Source: CAD feature listing. Evaluate the final solid. Frame: model axes, mm. A direction names the side the tool comes from. Give positions to 0.01 mm unless a question says otherwise; leave off trailing zeros. Loops run counter-clockwise (first coordinate to the right, second up) from the corner with the lowest first, then second, coordinate; pieces in that order, holes last. Notation, with made-up numbers: (40.5, -31.5) - (83.5, -31.5) arc R30 cw to (83.5, 4.5) - close; hole circle Ø1 at (-25.75, 28.5). An arc over 180 degrees is marked (long way). Put each result on its own line as item: value.
```python
from build123d import *

# Parameters (mm, degrees)
SKETCH_1_R          = 4.5
EXTRUDE_1_DEPTH     = 10
EXTRUDE_2_DEPTH     = 9
EXTRUDE_3_DEPTH     = 14
CUT_EXTRUDE_1_DEPTH = 29


with BuildPart() as part:
    # 草圖1 → 填料-伸長1 (new body)
    with BuildSketch(Plane.XY):
        with BuildLine():
            Line((-36, 9), (36, 9))
            ThreePointArc((36, 9), (45, 0), (36, -9))
            Line((36, -9), (-36, -9))
            ThreePointArc((-36, -9), (-45, 0), (-36, 9))
        make_face()
        with Locations((36, 0)):
            Circle(SKETCH_1_R, mode=Mode.SUBTRACT)
        with Locations((-36, 0)):
            Circle(SKETCH_1_R, mode=Mode.SUBTRACT)
    extrude(amount=EXTRUDE_1_DEPTH)

    # 草圖3 → 填料-伸長2 (add, symmetric)
    with BuildSketch(Plane(origin=(0, 0, 0), x_dir=(1, 0, 0), z_dir=(0, 1, 0))):
        with BuildLine():
            Line((-30, 0), (30, 0))
            ThreePointArc((30, 0), (0, -30), (-30, 0))
        make_face()
    extrude(amount=EXTRUDE_2_DEPTH, both=True)

    # 草圖4 → 填料-伸長3 (add, symmetric)
    with BuildSketch(Plane(origin=(0, 0, 0), x_dir=(1, 0, 0), z_dir=(0, 1, 0))):
        with BuildLine():
            Line((-24, 0), (24, 0))
            ThreePointArc((24, 0), (0, -24), (-24, 0))
        make_face()
    extrude(amount=EXTRUDE_3_DEPTH, both=True)

    # 草圖5 → 除料-伸長1 (cut, through all)
    with BuildSketch(Plane(origin=(0, 14, 0), x_dir=(1, 0, 0), z_dir=(0, 1, 0))):
        with BuildLine():
            Line((-18, 0), (18, 0))
            ThreePointArc((18, 0), (0, -18), (-18, 0))
        make_face()
    extrude(amount=-CUT_EXTRUDE_1_DEPTH, mode=Mode.SUBTRACT)


solid = part.part
```
1) Section query B-B, the plane y = 3.5. Output: boundary loops of the cut face in (x, z), plus the area to 3 significant figures.
Check result:
outline: (-44.29, 0) - (-38.83, 0) - (-38.83, 10) - (-44.29, 10) - close; (-33.17, 0) - (-18, 0) arc R18 cw to (18, 0) - (33.17, 0) - (33.17, 10) - (28.28, 10) arc R30 ccw to (-28.28, 10) - (-33.17, 10) - close; (38.83, 0) - (44.29, 0) - (44.29, 10) - (38.83, 10) - close
area: 1,090 mm²
2) Pin query (flat end, axial travel): P1, Ø8, axis at y = 9.5, z = 21.5, coming from the +X side; P2, Ø2, axis at x = -33.5, y = -9, coming from the +Z side; P3, Ø5, axis at x = -27, z = 7, coming from the -Y side. Return the tip coordinate at first contact, or that it passes through.
Check result:
P1: x = 24.34
P2: z = 10
P3: y = -9
3) Section query D-D, the plane x = 0. Output: boundary loops of the cut face in (y, z), plus the area to 3 significant figures.
Check result:
outline: (-14, 18) - (14, 18) - (14, 24) - (9, 24) - (9, 30) - (-9, 30) - (-9, 24) - (-14, 24) - close
area: 276 mm²
4) Section query C-C, the plane z = 14. Output: boundary loops of the cut face in (x, y), plus the area to 3 significant figures.
Check result:
outline: (-26.53, -9) - (-19.49, -9) - (-19.49, -14) - (-11.31, -14) - (-11.31, 14) - (-19.49, 14) - (-19.49, 9) - (-26.53, 9) - close; (11.31, -14) - (19.49, -14) - (19.49, -9) - (26.53, -9) - (26.53, 9) - (19.49, 9) - (19.49, 14) - (11.31, 14) - close
area: 711 mm²
5) Material intervals for line 1 along Y through (x, z) = (-36, 5); line 2 along X through (y, z) = (1.25, 8); line 3 along Z through (x, y) = (-35, 8), sorted ascending. Write a range as [from, to].
Check result:
line 1: [-9, -4.5], [4.5, 9]
line 2: [-44.91, -40.32], [-31.68, -16.12], [16.12, 31.68], [40.32, 44.91]
line 3: [0, 10]
6) Section query A-A, the plane x = -33. Output: boundary loops of the cut face in (y, z), plus the area to 3 significant figures.
Check result:
outline: (-9, 0) - (-3.35, 0) - (-3.35, 10) - (-9, 10) - close; (3.35, 0) - (9, 0) - (9, 10) - (3.35, 10) - close
area: 113 mm²
7) Access query for faces 1 (the flat face through (31, 0, 10)), 2 (the cylindrical face through (0.528, -11.465, 23.994)), 3 (the flat face through (0.1, -14, 18.2)), 4 (the flat face through (-40.2, 2.1, 10)), 5 (the cylindrical face through (0.528, 11.535, 23.994)). Directions: +Z, -Z, +X, -X, +Y, -Y. A direction counts if a zero-diameter tool reaches every point of the face in a straight line with its end or side. Return the directions, or none.
Check result:
face 1: +Z, +X, +Y, -Y
face 2: +Z, -Y
face 3: +Z, -Z, +X, -X, -Y
face 4: +Z, -X, +Y, -Y
face 5: +Z, +Y
8) Mould query, pull axis Y, two halves, no side actions, for faces 6 (the cylindrical face through (0, 0, 18)), 7 (the flat face through (0.1, 14, 18.2)), 8 (the cylindrical face through (-31.708, 1.352, 4.93)), 9 (the cylindrical face through (40.292, 1.352, 4.93)). Classes: pulls with the +Y half, pulls with the -Y half, needs draft (parallel to the pull), parting line crosses it, or undercut.
Check result:
face 6: needs draft
face 7: pulls with the +Y half
face 8: undercut
face 9: undercut
